Geometry check sheet. Reference: the model listing, model coordinates, mm. Give positions to 0.01 mm unless a question says otherwise; leave off trailing zeros. Order: outer loops, then holes, each group sorted by start corner. A loop starts at its lowest first (then second) coordinate and runs counter-clockwise, first axis right, second up. Notation, with made-up numbers: M 9.5,22.25 L 27.5,22.25 A18 cw 27.5,50.25 Z; hole C -27.5,-13 d1. An arc over 180 degrees is marked long. Answer as CSV lines item,"result".
from build123d import *

# Parameters (mm, degrees)
F1_DEPTH = 100


with BuildPart() as f1:
    # F0 (on Top) → F1 (new body)
    with BuildSketch(Plane.XY):
        Polygon((-11.8646007031, -21.5996578336), (-33.768478781, 10.9519390389), (-45.1385089955, -11.7881209321), align=None)
        Polygon((12.1688209474, 18.2532314211), (-41.6782125831, 32.8558161855), (-33.768478781, 10.9519390389), (1.2571312237, 0.1591635659), align=None)
        Polygon((17.9066221318, -4.9712029599), (12.1688209474, 18.2532314211), (1.2571312237, 0.1591635659), align=None)
        Polygon((-45.1385089955, -11.7881209321), (-59.3230053782, -7.6055130921), (-56.8892396986, -35.2895818651), align=None)
        Polygon((-33.768478781, 10.9519390389), (-41.6782125831, 32.8558161855), (-59.3230053782, -7.6055130921), (-45.1385089955, -11.7881209321), align=None)
        Polygon((1.2571312237, 0.1591635659), (-33.768478781, 10.9519390389), (-11.8646007031, -21.5996578336), align=None)
        Polygon((17.9066221318, -4.9712029599), (1.2571312237, 0.1591635659), (-11.8646007031, -21.5996578336), (-45.1385089955, -11.7881209321), (-56.8892396986, -35.2895818651), (-11.8646007031, -51.1090494692), (18.1195368493, -5.8330006636), align=None)
    extrude(amount=F1_DEPTH)


solid = f1.part
(1) Material ranges on line 1 (Y direction, x = -11, z = 68); line 2 (X direction, y = -31.5, z = 80.5); line 3 (X direction, y = -1, z = 32.5), recorded low to high.
The answers:
line 1,"y = -49.8 to 24.54"
line 2,"x = -57.22 to 1.12"
line 3,"x = -56.44 to 16.93"
(2) Section check A-A on z = 56. Enter the section's corners in (x, y), then the cut area to 3 significant figures.
The answers:
outline,"M -59.32,-7.61 L -56.89,-35.29 L -11.86,-51.11 L 18.12,-5.83 L 12.17,18.25 L -41.68,32.86 Z"
area,"4,490 mm2"
(3) Section check B-B on y = -27. Enter the section's corners in (x, z), then the cut area to 3 significant figures.
The answers:
outline,"M -57.62,0 L 4.1,0 L 4.1,100 L -57.62,100 Z"
area,"6,170 mm2"
(4) Gauge pin test, flat ends, axial feed: P1, Ø3, axis at x = -9.5, z = 74, coming from the -Y side; P2, Ø12, axis at x = -49, z = 63.5, coming from the -Y side; P3, Ø8, axis at y = -29, z = 86, coming from the +X side. Record the tip position at first contact, or that the pin passes through.
The answers:
P1,"stops at y = -49.8"
P2,"stops at y = -40.17"
P3,"stops at x = 5.43"
(5) Section check C-C on x = -9.5. Enter the section's corners in (y, z), then the cut area to 3 significant figures.
The answers:
outline,"M -47.54,0 L 24.13,0 L 24.13,100 L -47.54,100 Z"
area,"7,170 mm2"
